```python
from build123d import *

# Parameters (mm, degrees)
ESBO_O1_W                  = 115.09677689
ESBO_O1_H                  = 63
RESSALTO_EXTRUS_O1_DEPTH   = 2
ESBO_O5_R                  = 2
CORTE_EXTRUS_O3_DEPTH      = 66.635866816
FILETE1_R                  = 3
CORTE_EXTRUS_O4_DEPTH      = 66.635866816
CORTE_EXTRUS_O4_DEPTH_BACK = 66.635866816
ESBO_O6_W                  = 7
ESBO_O6_H                  = 9


with BuildPart() as part:
    # Esboço1 → Ressalto-extrusão1 (new body)
    with BuildSketch(Plane(origin=(0, 0, 0), x_dir=(1, 0, 0), z_dir=(0, 1, 0))):
        Rectangle(ESBO_O1_W, ESBO_O1_H)
    extrude(amount=RESSALTO_EXTRUS_O1_DEPTH)

    # Esboço5 → Corte-extrusão3 (cut, through all)
    with BuildSketch(Plane(origin=(0, 2, 0), x_dir=(1, 0, 0), z_dir=(0, 1, 0))):
        with Locations(Location((53.548388445, 27.5, 0), (0, 0, 270))):
            Circle(ESBO_O5_R)
        with Locations(Location((53.548388445, -27.5, 0), (0, 0, 90))):
            Circle(ESBO_O5_R)
        with Locations(Location((-53.548388445, -27.5, 0), (0, 0, 270))):
            Circle(ESBO_O5_R)
        with Locations(Location((-53.548388445, 27.5, 0), (0, 0, 90))):
            Circle(ESBO_O5_R)
    extrude(amount=-CORTE_EXTRUS_O3_DEPTH, mode=Mode.SUBTRACT)

    # Filete1
    filete1_edges = [part.edges().sort_by_distance(p)[0] for p in [
        (-57.548388445, 1, -31.5),
        (57.548388445, 1, -31.5),
        (57.548388445, 1, 31.5),
        (-57.548388445, 1, 31.5),
    ]]
    fillet(filete1_edges, radius=FILETE1_R)

    # Esboço6 → Corte-extrusão4 (cut, two sides: drawn at the far end of the back side and taken through both)
    with BuildSketch(Plane(origin=(0, 2, 0), x_dir=(1, 0, 0), z_dir=(0, 1, 0)).offset(-CORTE_EXTRUS_O4_DEPTH_BACK)):
        with Locations((-39.048388445, 0)):
            Rectangle(ESBO_O6_W, ESBO_O6_H)
        with Locations((39.048388445, 0)):
            Rectangle(ESBO_O6_W, ESBO_O6_H)
    extrude(amount=CORTE_EXTRUS_O4_DEPTH + CORTE_EXTRUS_O4_DEPTH_BACK, mode=Mode.SUBTRACT)


solid = part.part
```
Build history of the part. All positions in model axes, mm. A direction names the side the tool comes from. Give positions to 0.01 mm unless a question says otherwise; leave off trailing zeros. Loops run counter-clockwise (first coordinate to the right, second up) from the corner with the lowest first, then second, coordinate; pieces in that order, holes last.
Item 1: Flat gauge pins, fed straight in: pin 1 (8 mm diameter, centred on x = 1.5, z = 14.5, fed in from -Y); pin 2 (2.5 mm diameter, centred on x = -53.55, z = -27.5, fed in from +Y). Where does each tip first touch, or does it go through?
Answers follow:
pin 1: stops at y = 0
pin 2: passes through
Item 2: Pull direction Z, two halves, no side cores. Call faces 3 (the face through (-1, 1, -31.5)), 4 (the face through (-56.69, 1.01, 30.6)), 5 (the face through (35.548, 1, 0)), 6 (the face through (-57.548, 1, 0)): released by +Z, released by -Z, zero draft, split by the parting line, or undercut.
Answers follow:
face 3: released by -Z
face 4: released by +Z
face 5: undercut
face 6: zero draft
Item 3: Slice it at B-B, the plane y = 0.65. List the corners of the cut face in (x, z).
Answers follow:
outline: (-57.55, -28.5) arc R3 ccw to (-54.55, -31.5) - (54.55, -31.5) arc R3 ccw to (57.55, -28.5) - (57.55, 28.5) arc R3 ccw to (54.55, 31.5) - (-54.55, 31.5) arc R3 ccw to (-57.55, 28.5) - close; hole circle Ø4 at (-53.55, -27.5); hole circle Ø4 at (-53.55, 27.5); hole (-42.55, -4.5) - (-35.55, -4.5) - (-35.55, 4.5) - (-42.55, 4.5) - close; hole (35.55, -4.5) - (42.55, -4.5) - (42.55, 4.5) - (35.55, 4.5) - close; hole circle Ø4 at (53.55, -27.5); hole circle Ø4 at (53.55, 27.5)
Item 4: Drill centre lines: line 1 (X direction, y = 0.95, z = 27.5); line 2 (X direction, y = 1.75, z = -28); line 3 (Z direction, x = -41, y = 0.35). Where is each one in solid material? Low to high.
Answers follow:
line 1: x = -57.55 to -55.55, -51.55 to 51.55, 55.55 to 57.55
line 2: x = -57.55 to -55.48, -51.61 to 51.61, 55.48 to 57.55
line 3: z = -31.5 to -4.5, 4.5 to 31.5
Item 5: Slice it at A-A, the plane z = 0. List the corners of the cut face in (x, y), and give its area (3 significant figures).
Answers follow:
outline: (-57.55, 0) - (-42.55, 0) - (-42.55, 2) - (-57.55, 2) - close; (-35.55, 0) - (35.55, 0) - (35.55, 2) - (-35.55, 2) - close; (42.55, 0) - (57.55, 0) - (57.55, 2) - (42.55, 2) - close
area: 202 mm2
Item 6: Which spindle directions (+Z, -Z, +X, -X, +Y, -Y) get a long thin tool onto all of the face, cutting with end or side? Do faces 1 (the face through (-56.69, 1.01, -30.6)), 2 (the face through (-42.548, 1, 0)). Say none if no direction does.
Answers follow:
face 1: -Z, -X, +Y, -Y
face 2: +Y, -Y
